Geometry check sheet. Reference: the model listing, model coordinates, mm. Round coordinates to 2 decimals unless told otherwise and drop trailing zeros. Loops run counter-clockwise (first coordinate to the right, second up) from the corner with the lowest first, then second, coordinate; pieces in that order, holes last. Notation, with made-up numbers: M -16.75,19 L 15.25,19 A11 ccw 15.25,29 Z; hole C -24.5,36 d8. An arc over 180 degrees is marked long. Use one line per item in the form item = value. Start each with the question number.
1. Cross-section at A-A (x = 440.5). Record the boundary of the cut face in (y, z), then the cut area to 3 significant figures.
2. Go/stop test with flat-tipped pins: pin 1 (5 mm diameter, centred on x = 356, z = 16.5, fed in from -Y); pin 2 (2.5 mm diameter, centred on x = 242, y = -102.5, fed in from -Z). Record where each tip stops, or that it passes through.
3. Material ranges on line 1 (Y direction, x = 424, z = 15.5); line 2 (Y direction, x = 191, z = 27.25); line 3 (Y direction, x = 200, z = 28.5), recorded low to high.
```python
from build123d import *

# Parameters (mm, degrees)
F1_DEPTH  = 862
F1_FACE_W = 862
F1_FACE_H = 6
F2_DEPTH  = 1


with BuildPart() as f1:
    # F0 (on Right) → F1 (new body)
    with BuildSketch(Plane.YZ):
        with BuildLine():
            Line((117.323911, 35.13468), (-115.676089, 35.13468))
            ThreePointArc((-115.676089, 35.13468), (-121.332944, 32.791535), (-123.676089, 27.13468))
            Line((-123.676089, 27.13468), (-123.676089, 21.13468))
            ThreePointArc((-123.676089, 21.13468), (-121.332944, 15.477826), (-115.676089, 13.13468))
            Line((-115.676089, 13.13468), (-107.676089, 13.13468))
            Line((-107.676089, 13.13468), (-107.676089, 19.13468))
            Line((-107.676089, 19.13468), (-97.676089, 19.13468))
            Line((-97.676089, 19.13468), (-97.676089, 13.13468))
            Line((-97.676089, 13.13468), (117.323911, 13.13468))
            Line((117.323911, 13.13468), (117.323911, 35.13468))
        make_face()
    extrude(amount=F1_DEPTH)

    # F1_face (on face) → F2 (join)
    with BuildSketch(Plane(origin=(431, -97.676089, 16.13468), x_dir=(1, 0, 0), z_dir=(0, -1, 0))):
        Rectangle(F1_FACE_W, F1_FACE_H)
    extrude(amount=F2_DEPTH)


solid = f1.part
```
Reported:
q1.outline = M -123.68,21.13 A8 ccw -115.68,13.13 L -107.68,13.13 L -107.68,19.13 L -98.68,19.13 L -98.68,13.13 L 117.32,13.13 L 117.32,35.13 L -115.68,35.13 A8 ccw -123.68,27.13 Z
q1.area = 5,220 mm²
q2.pin_1 = -123.39
q2.pin_2 = 19.13
q3.line_1 = -121.36 to -107.68, -98.68 to 117.32
q3.line_2 = -123.68 to 117.32
q3.line_3 = -123.56 to 117.32
